```python
from build123d import *

# Parameters (mm, degrees)
F1_DEPTH = 22.225
F2_W     = 4.318
F2_H     = 12.7
F3_DEPTH = 11.212402643
F4_R     = 2.15899
F5_R     = 3.175
F6_DEPTH = 3.81
F8_DEPTH = 25.4
F9_R     = 3.81


# Not quite as in the source:
# - a fillet or chamfer is up to 0.001 mm smaller than in the source, because OpenCascade refuses the exact size


with BuildPart() as f1:
    # F0 (on Front) → F1 (new body)
    with BuildSketch(Plane.XZ):
        Polygon((11.5514947486, -84.959096284), (2.8641831082, -61.090903716), (0, -62.1333811129), (8.6873116405, -86.0015736808), align=None)
    extrude(amount=F1_DEPTH)

    # F2 (on face) → F3 (cut, through all)
    with BuildSketch(Plane(origin=(-19.9692837636, 0, -7.2682248896), x_dir=(0, -1, 0), z_dir=(-0.9396926208, 0, -0.3420201433))):
        with Locations((11.1125, -71.0862797362)):
            Rectangle(F2_W, F2_H)
        with Locations((11.1125, -93.3112797362)):
            Rectangle(F2_W, F2_H)
    extrude(amount=-F3_DEPTH, mode=Mode.SUBTRACT)

    # F4 (radius 2.159 in the source; OpenCascade refuses exactly that, so slightly less here)
    f4_edges = [f1.edges().sort_by_distance(p)[0] for p in [
        (3.603919, -8.9535, -67.579191),
        (3.603919, -13.2715, -67.579191),
        (7.947575, -13.2715, -79.513287),
        (7.947575, -8.9535, -79.513287),
    ]]
    fillet(f4_edges, radius=F4_R)

    # F5 (on Front) → F6 (join)
    with BuildSketch(Plane.XZ):
        Polygon((11.5514947486, -84.959096284), (2.8641831082, -61.090903716), (-13.1392344849, -61.090903716), (-26.1296610716, -25.4), (-64.2296610716, -25.4), (-64.2296610716, -84.959096284), align=None)
        with Locations((-51.5296610716, -38.1)):
            Circle(F5_R, mode=Mode.SUBTRACT)
    extrude(amount=-F6_DEPTH)

    # F7 (on Front) → F8 (cut)
    with BuildSketch(Plane.XZ):
        Polygon((-65.5156196266, -25.4), (-51.5296610716, -39.3859585549), (-38.8296610716, -26.6859585549), (-38.8296610716, -25.4), align=None)
    extrude(amount=-F8_DEPTH, mode=Mode.SUBTRACT)

    # F9
    f9_edges = [f1.edges().sort_by_distance(p)[0] for p in [
        (-64.229661, 1.905, -26.685959),
    ]]
    fillet(f9_edges, radius=F9_R)


solid = f1.part
```
The model under review builds one solid part; all positions refer to its coordinate system, in mm. A direction names the side the tool comes from. Round coordinates to 2 decimals unless told otherwise and drop trailing zeros. Order: outer loops, then holes, each group sorted by start corner. A loop starts at its lowest first (then second) coordinate and runs counter-clockwise, first axis right, second up. Notation, with made-up numbers: (46, 55.5) -> (104, 55.5) arc R18 ccw to (104, 67.5) -> close; hole circle Ø8 at (-39, 60.5). An arc over 180 degrees is marked (long way). One line per item, written item: value. Start each with the question number.
Q1. Machinability: for faces 1 (the face through (1.452, -10.957, -61.605)), 2 (the face through (7.757, -9.603, -78.927)), 3 (the face through (-5, 2, -61.091)), 4 (the face through (3.846, -12.656, -68.182)), which of the approach directions +Z, -Z, +X, -X, +Y, -Y give a long, thin tool a straight path to every point of the face, cutting with its end or side? Answer none if there is none.
Q2. Mouldability with a two-part tool opening along Y and no side actions: class faces 5 (the face through (6, -22.225, -74)), 6 (the face through (3.835, -9.603, -68.15)), 7 (the face through (4.283, -8.487, -73.9)) as released by +Y, released by -Y, zero draft, split by the parting line, or undercut.
Q3. Take a section at C-C (z = -38.1). Write out the cut boundary in (x, y).
Q4. Take a section at A-A (z = -75). Write out the cut boundary in (x, y) (1 decimal).
Q5. Clearance check with flat-ended pins moving along their axes: pin 1 Ø10 at (x, y) = (-24, -4.5) entering from -Z; pin 2 Ø5 at (x, z) = (-21, -51) entering from -Y; pin 3 Ø2 at (x, y) = (-19.5, -2) entering from -Z; pin 4 Ø0.5 at (x, z) = (10, -85.5) entering from +Y. State where each tip first meets the part, or that it passes through.
Q6. Take a section at D-D (x = -32.5). Write out the cut boundary in (y, z).
Q7. Wall thickness on line 1 (Y direction, x = -35.5, z = -83); line 2 (X direction, y = 2.3, z = -38.1); line 3 (Z direction, x = -60.5, y = 2): over which ranges is each line inside the solid? List them lowest first.
Reported:
1. face 1: +Z, -X, -Y
1. face 2: +Z, -X
1. face 3: +Z, +X, +Y, -Y
1. face 4: -Z, +X
2. face 5: released by -Y
2. face 6: undercut
2. face 7: zero draft
3. outline: (-64.23, 0) -> (-54.7, 0) -> (-54.7, 3.81) -> (-64.23, 3.81) -> close; (-48.35, 0) -> (-21.51, 0) -> (-21.51, 3.81) -> (-48.35, 3.81) -> close
4. outline: (-64.2, 0) -> (4.7, 0) -> (4.7, -9) -> (7.9, -9) -> (7.9, 3.8) -> (-64.2, 3.8) -> close; (4.7, -22.2) -> (7.9, -22.2) -> (7.9, -13.3) -> (4.7, -13.3) -> close
5. pin 1: stops at z = -84.96
5. pin 2: stops at y = 0
5. pin 3: passes through
5. pin 4: stops at y = 0
6. outline: (0, -84.96) -> (3.81, -84.96) -> (3.81, -25.4) -> (0, -25.4) -> close
7. line 1: y = 0 to 3.81
7. line 2: x = -64.23 to -54.7, -48.35 to -21.51
7. line 3: z = -84.96 to -32.07
